from build123d import *

# Parameters (mm, degrees)
F0_W      = 90
F0_H      = 90
F1_DEPTH  = 5
F2_W      = 15
F2_H      = 30
F3_ANGLE  = 2
F4_W      = 15
F4_H      = 30
F5_ANGLE  = -4
F6_W      = 15
F6_H      = 30
F7_ANGLE  = -6
F8_W      = 15
F8_H      = 30
F9_ANGLE  = -8
F10_W     = 15
F10_H     = 30
F11_ANGLE = -10
F12_W     = 15
F12_H     = 30
F13_ANGLE = -12
F14_W     = 15
F14_H     = 30
F15_ANGLE = -14
F16_W     = 15
F16_H     = 30
F17_ANGLE = -16
F18_W     = 15
F18_H     = 30
F19_ANGLE = -18
F20_W     = 15
F20_H     = 30
F21_ANGLE = -20
F22_W     = 15
F22_H     = 30
F23_ANGLE = -25
F24_W     = 15
F24_H     = 30
F25_ANGLE = -30
F26_W     = 15
F26_H     = 30
F27_ANGLE = -35
F28_W     = 15
F28_H     = 30
F29_ANGLE = -40
F30_W     = 15
F30_H     = 30
F31_ANGLE = -45
F32_W     = 15
F32_H     = 30
F33_ANGLE = -50
F34_W     = 15
F34_H     = 30
F35_ANGLE = -55


with BuildPart() as f1:
    # F0 (on Top) → F1 (new body)
    with BuildSketch(Plane.XY):
        Rectangle(F0_W, F0_H)
    extrude(amount=F1_DEPTH)

    # F2 (on Top) → F3 (revolve)
    with BuildSketch(Plane.XY):
        with Locations((22.5, 30)):
            Rectangle(F2_W, F2_H)
    revolve(axis=Axis((22.5, 45, 0), (1, 0, 0)), revolution_arc=F3_ANGLE)

    # F4 (on Top) → F5 (revolve)
    with BuildSketch(Plane.XY):
        with Locations((7.5, 30)):
            Rectangle(F4_W, F4_H)
    revolve(axis=Axis((7.5, 45, 0), (-1, 0, 0)), revolution_arc=F5_ANGLE)

    # F6 (on Top) → F7 (revolve)
    with BuildSketch(Plane.XY):
        with Locations((-7.5, 30)):
            Rectangle(F6_W, F6_H)
    revolve(axis=Axis((-7.5, 45, 0), (-1, 0, 0)), revolution_arc=F7_ANGLE)

    # F8 (on Top) → F9 (revolve)
    with BuildSketch(Plane.XY):
        with Locations((-22.5, 30)):
            Rectangle(F8_W, F8_H)
    revolve(axis=Axis((-22.5, 45, 0), (-1, 0, 0)), revolution_arc=F9_ANGLE)

    # F10 (on Top) → F11 (revolve)
    with BuildSketch(Plane.XY):
        with Locations((-37.5, 30)):
            Rectangle(F10_W, F10_H)
    revolve(axis=Axis((-37.5, 45, 0), (-1, 0, 0)), revolution_arc=F11_ANGLE)

    # F12 (on Top) → F13 (revolve)
    with BuildSketch(Plane.XY):
        with Locations((37.5, 0)):
            Rectangle(F12_W, F12_H)
    revolve(axis=Axis((37.5, 15, 0), (-1, 0, 0)), revolution_arc=F13_ANGLE)

    # F14 (on Top) → F15 (revolve)
    with BuildSketch(Plane.XY):
        with Locations((22.5, 0)):
            Rectangle(F14_W, F14_H)
    revolve(axis=Axis((22.5, 15, 0), (-1, 0, 0)), revolution_arc=F15_ANGLE)

    # F16 (on Top) → F17 (revolve)
    with BuildSketch(Plane.XY):
        with Locations((7.5, 0)):
            Rectangle(F16_W, F16_H)
    revolve(axis=Axis((7.5, 15, 0), (-1, 0, 0)), revolution_arc=F17_ANGLE)

    # F18 (on Top) → F19 (revolve)
    with BuildSketch(Plane.XY):
        with Locations((-7.5, 0)):
            Rectangle(F18_W, F18_H)
    revolve(axis=Axis((-7.5, 15, 0), (-1, 0, 0)), revolution_arc=F19_ANGLE)

    # F20 (on Top) → F21 (revolve)
    with BuildSketch(Plane.XY):
        with Locations((-22.5, 0)):
            Rectangle(F20_W, F20_H)
    revolve(axis=Axis((-22.5, 15, 0), (-1, 0, 0)), revolution_arc=F21_ANGLE)

    # F22 (on Top) → F23 (revolve)
    with BuildSketch(Plane.XY):
        with Locations((-37.5, 0)):
            Rectangle(F22_W, F22_H)
    revolve(axis=Axis((-37.5, 15, 0), (-1, 0, 0)), revolution_arc=F23_ANGLE)

    # F24 (on Top) → F25 (revolve)
    with BuildSketch(Plane.XY):
        with Locations((37.5, -30)):
            Rectangle(F24_W, F24_H)
    revolve(axis=Axis((37.5, -15, 0), (-1, 0, 0)), revolution_arc=F25_ANGLE)

    # F26 (on Top) → F27 (revolve)
    with BuildSketch(Plane.XY):
        with Locations((22.5, -30)):
            Rectangle(F26_W, F26_H)
    revolve(axis=Axis((22.5, -15, 0), (-1, 0, 0)), revolution_arc=F27_ANGLE)

    # F28 (on Top) → F29 (revolve)
    with BuildSketch(Plane.XY):
        with Locations((7.5, -30)):
            Rectangle(F28_W, F28_H)
    revolve(axis=Axis((7.5, -15, 0), (-1, 0, 0)), revolution_arc=F29_ANGLE)

    # F30 (on Top) → F31 (revolve)
    with BuildSketch(Plane.XY):
        with Locations((-7.5, -30)):
            Rectangle(F30_W, F30_H)
    revolve(axis=Axis((-7.5, -15, 0), (-1, 0, 0)), revolution_arc=F31_ANGLE)

    # F32 (on Top) → F33 (revolve)
    with BuildSketch(Plane.XY):
        with Locations((-22.5, -30)):
            Rectangle(F32_W, F32_H)
    revolve(axis=Axis((-22.5, -15, 0), (-1, 0, 0)), revolution_arc=F33_ANGLE)

    # F34 (on Top) → F35 (revolve)
    with BuildSketch(Plane.XY):
        with Locations((-37.5, -30)):
            Rectangle(F34_W, F34_H)
    revolve(axis=Axis((-37.5, -15, 0), (-1, 0, 0)), revolution_arc=F35_ANGLE)


solid = f1.part
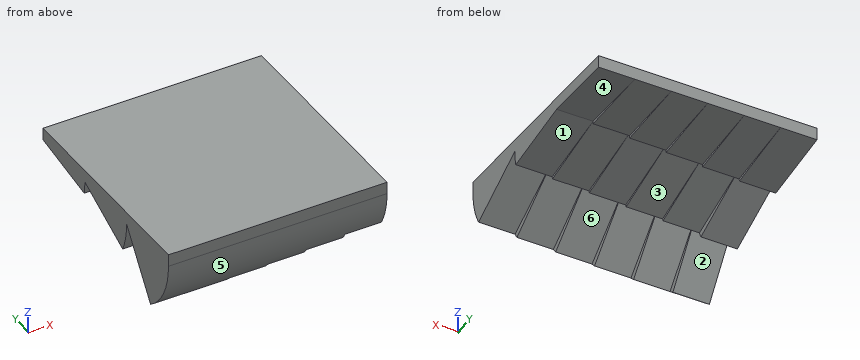
Geometry: final body of the model. Coordinates: model frame, mm. Face numbers are marked on the shaded views. A direction names the side the tool comes from. Give positions to 0.01 mm unless a question says otherwise; leave off trailing zeros. Write each loop counter-clockwise with the first axis right and the second up, starting at its lowest first coordinate (ties: lowest second). Pieces come first, ordered by that corner, then holes. Notation, with made-up numbers: (73.5, 14) -> (96.5, 14) arc R6 cw to (96.5, 20) -> close; hole circle Ø7 at (45.25, -27). An arc over 180 degrees is marked (long way). Answer in a Markdown table with one row per item.
(1) Set-up query: the marked faces 1, 2 and 3. Return all of +Z, -Z, +X, -X, +Y, -Y with unobstructed straight access to the full face (end or side cutting, diameter ignored); none if empty.
Answers below:
| item | result |
|---|---|
| face 1 | -Z, +X, +Y |
| face 2 | -Z, +X, -X |
| face 3 | -Z, +X |
(2) Section query D-D on y = 21.5. Return loops of the section in (x, z).
Answers below:
| item | result |
|---|---|
| outline | (-45, -4.14) -> (-30, -4.14) -> (-30, -3.3) -> (-15, -3.3) -> (-15, -2.47) -> (0, -2.47) -> (0, -1.64) -> (15, -1.64) -> (15, -0.82) -> (30, -0.82) -> (30, 0) -> (45, 0) -> (45, 5) -> (-45, 5) -> close |
(3) Section query A-A on x = -26.5. Return loops of the section in (y, z), then the cut area to 3 significant figures.
Answers below:
| item | result |
|---|---|
| outline | (-45, 0) arc R30 ccw to (-34.28, -22.98) -> (-15, 0) arc R30 ccw to (-13.19, -10.26) -> (15, 0) arc R30 ccw to (15.29, -4.18) -> (45, 0) -> (45, 5) -> (-45, 5) -> close |
| area | 1,060 mm^2 |
(4) Draft query along Y for the marked faces 4, 5 and 6. Return one class per face: +Y half, -Y half, draft (parallel to the pull), parting line (faces both ways), or undercut.
Answers below:
| item | result |
|---|---|
| face 4 | draft |
| face 5 | -Y half |
| face 6 | undercut |
(5) Pin query (flat end, axial travel): pin 1 (6.5 mm diameter, centred on y = -22.5, z = -14.5, fed in from +X); pin 2 (12 mm diameter, centred on x = 37.5, y = 24.5, fed in from -Z); pin 3 (4 mm diameter, centred on y = -30, z = -12, fed in from +X). Return the tip coordinate at first contact, or that it passes through.
Answers below:
| item | result |
|---|---|
| pin 1 | x = -30 |
| pin 2 | z = 0 |
| pin 3 | x = 30 |
(6) Ray query, line 1 along Z through (x, y) = (39, 30); line 2 along X through (y, z) = (-36.5, -17.25); line 3 along X through (y, z) = (-6, -7.5). Return the intervals inside material, ascending. Write a range as [from, to].
Answers below:
| item | result |
|---|---|
| line 1 | [0, 5] |
| line 2 | [-45, 15] |
| line 3 | [-45, -15] |
(7) Section query C-C on x = 6. Return loops of the section in (y, z), then the cut area to 3 significant figures.
Answers below:
| item | result |
|---|---|
| outline | (-45, 0) arc R30 ccw to (-37.98, -19.28) -> (-15, 0) arc R30 ccw to (-13.84, -8.27) -> (15, 0) arc R30 ccw to (15.07, -2.09) -> (45, 0) -> (45, 5) -> (-45, 5) -> close |
| area | 921 mm^2 |
(8) Section query B-B on y = 8.5. Return loops of the section in (x, z).
Answers below:
| item | result |
|---|---|
| outline | (-45, -3.03) -> (-30, -3.03) -> (-30, -2.37) -> (-15, -2.37) -> (-15, -2.11) -> (0, -2.11) -> (0, -1.86) -> (15, -1.86) -> (15, -1.62) -> (30, -1.62) -> (30, -1.38) -> (45, -1.38) -> (45, 5) -> (-45, 5) -> close |
